Autodesk Fusion 360 part; units mm, degrees
sketch "Sketch1" plane through (0, 0, 0) normal (0, 1, 0) x (1, 0, 0)
  circle A0 centre (0, 0) radius 75
  dimension "d1" = 150
extrude "Extrude1" add sketch "Sketch1" along normal blind 40 makes body 1
sketch "Sketch2" plane through (0, 40, 0) normal (0, 1, 0) x (-1, 0, 0)
  circle A0 centre (0, 0) radius 75
  circle A1 centre (0, 0) radius 55
  dimension "d4" = 110
extrude "Extrude2" add sketch "Sketch2" along normal blind 20 contours A1 bodies 1
sketch "Sketch3" plane through (0, 60, 0) normal (0, 1, 0) x (-1, 0, 0)
  circle A0 centre (0, 0) radius 55
sketch "Sketch4" plane through (0, 60, 0) normal (0, 1, 0) x (-1, 0, 0)
  circle A0 centre (0, 0) radius 10
  dimension "d7" = 20
extrude "Extrude3" cut sketch "Sketch4" against normal blind 10 bodies 1
sketch "Sketch6" plane through (0, 0, 0) normal (0, -1, 0) x (1, 0, 0)
  circle A0 centre (0, 0) radius 75
  circle A1 centre (0, 0) radius 12.5
  dimension "d10" = 25
extrude "Extrude4" cut sketch "Sketch6" against normal blind 30 contours A1 bodies 1
copy_body "Body->Comp1" bodies 1 removing the originals makes body 2 in component "Component"
component "Component" placed x (1, 0, 0) y (0, 1, 0) z (0, 0, 1) at (0, 0, 0)
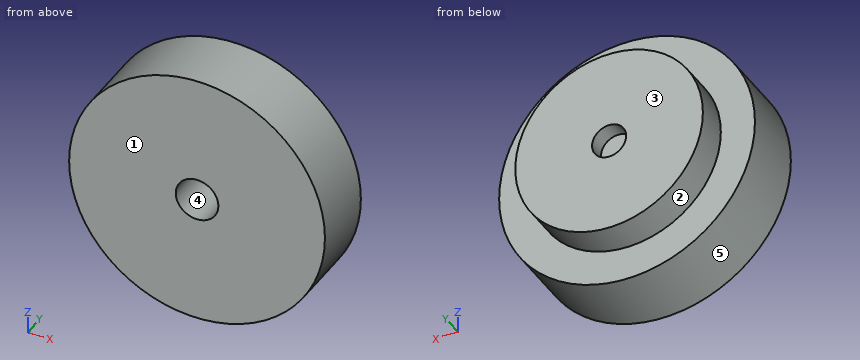
Part model, mm, in its own coordinate system. Face numbers are marked on the shaded views. A direction names the side the tool comes from. Round coordinates to 2 decimals unless told otherwise and drop trailing zeros. Write each loop counter-clockwise with the first axis right and the second up, starting at its lowest first coordinate (ties: lowest second). Pieces come first, ordered by that corner, then holes. Notation, with made-up numbers: M -7,14.5 L 45,14.5 A25 cw 45,32.5 Z; hole C 74,-15.5 d7. An arc over 180 degrees is marked long. One line per question, with ' | ' between items.
(1) Pin check, flat tips, straight feed: pin 1 (5 mm diameter, centred on y = 16, z = -7, fed in from +X); pin 2 (1 mm diameter, centred on y = 39, z = -59, fed in from -X); pin 3 (1 mm diameter, centred on x = -21, y = 8, fed in from -Z). Stop position of each tip, or through.
Answer key:
pin 1: stops at x = 74.86 | pin 2: stops at x = -46.93 | pin 3: stops at z = -72.14
(2) Saw through at C-C on z = 0. Write the cut outline in (x, y), then the cut area to 3 significant figures.
Answer key:
outline: M -75,0 L -12.5,0 L -12.5,30 L 12.5,30 L 12.5,0 L 75,0 L 75,40 L 55,40 L 55,60 L 10,60 L 10,50 L -10,50 L -10,60 L -55,60 L -55,40 L -75,40 Z | area: 7,250 mm^2
(3) Probe line 1 along Z through (x, y) = (0, 7); line 2 along Z through (x, y) = (0, 56.75); line 3 along Y through (x, z) = (-27.5, 62). List the from-to ranges inside material, lowest first.
Answer key:
line 1: z = -75 to -12.5, 12.5 to 75 | line 2: z = -55 to -10, 10 to 55 | line 3: y = 0 to 40
(4) 3-axis set-ups, long thin cutter, end or side, ignore diameter. For the marked faces 1 and 2: which of +Z, -Z, +X, -X, +Y, -Y reach the whole face in a straight line?
Answer key:
face 1: +Z, -Z, +X, -X, -Y | face 2: +Y
(5) Saw through at D-D on x = -15. Write the cut outline in (y, z).
Answer key:
outline: M 0,-73.48 L 40,-73.48 L 40,-52.92 L 60,-52.92 L 60,52.92 L 40,52.92 L 40,73.48 L 0,73.48 Z
(6) Two-plate mould, pull along X, no slides. Class the marked faces 3, 4 and 5: released by +X, released by -X, zero draft, split by the parting line, or undercut.
Answer key:
face 3: zero draft | face 4: undercut | face 5: split by the parting line
(7) Saw through at B-B on y = 19.5. Write the cut outline in (x, z).
Answer key:
outline: C 0,0 d150; hole C 0,0 d25
(8) Saw through at A-A on x = 0. Write the cut outline in (y, z), then the cut area to 3 significant figures.
Answer key:
outline: M 0,-75 L 40,-75 L 40,-55 L 60,-55 L 60,-10 L 50,-10 L 50,10 L 60,10 L 60,55 L 40,55 L 40,75 L 0,75 L 0,12.5 L 30,12.5 L 30,-12.5 L 0,-12.5 Z | area: 7,250 mm^2
